Geometry: see drawing. Coordinates: mm, zero at the bounding-box minimum. Coordinates: 2 decimals unless noted, no trailing zeros. Order: outer loops, then holes, each group sorted by start corner. A loop starts at its lowest first (then second) coordinate and runs counter-clockwise, first axis right, second up. Notation, with made-up numbers: (21.5, 3) - (54.5, 3) arc R11 ccw to (54.5, 19) - close; hole circle Ø3 at (11, 8). An arc over 180 degrees is marked (long way). Use a Markdown table: item, result. Add a question column.
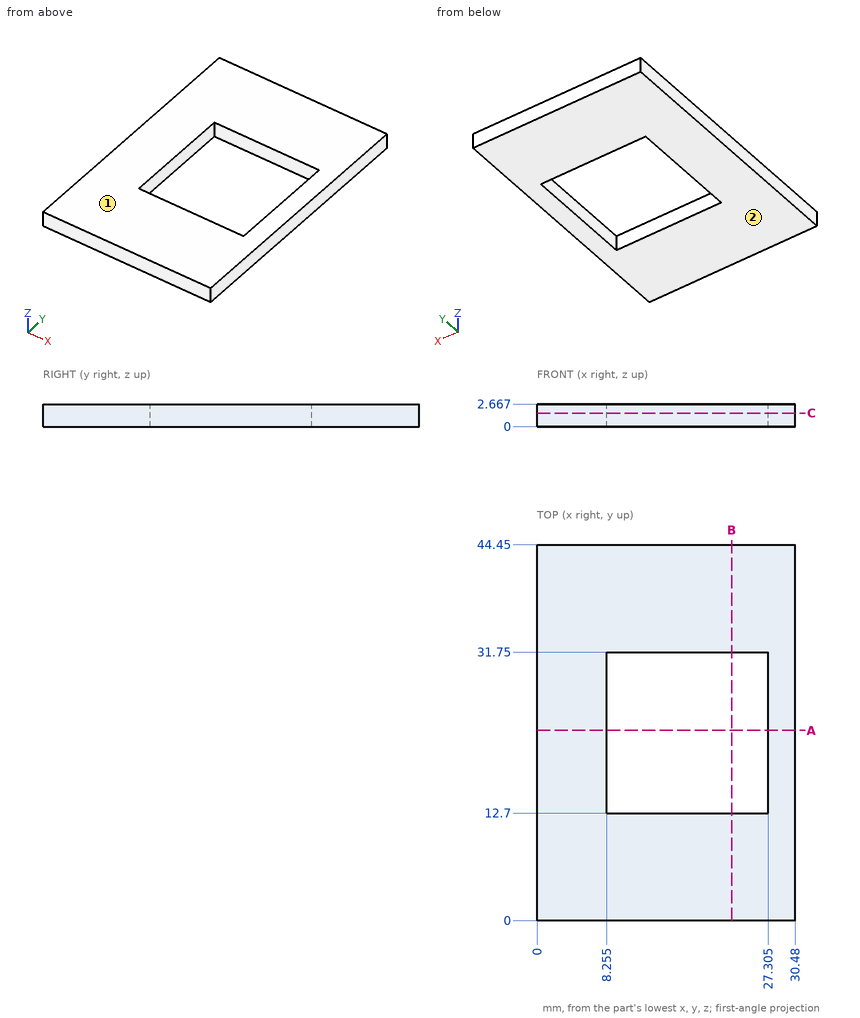
1) Section query B-B (x = 23). Return the cut outline in (y, z).
2) Line query: line 1 (Y direction, x = 14, z = 1); line 2 (X direction, y = 22, z = 1.8) (3 decimals). Output: solid intervals per line, ascending. Write a range as from..to.
3) Section query C-C (z = 1.6). Return the cut outline in (x, y) (3 decimals).
4) Section query A-A (y = 22.5). Return the cut outline in (x, z) (3 decimals), and give its area (3 significant figures).
5) Draft query along Z for the marked faces 1 and 2. Return one class per face: released by +Z, released by -Z, zero draft, split by the parting line, or undercut.
From the geometry:
| question | item | result |
|---|---|---|
| 1 | outline | (0, 0) - (12.7, 0) - (12.7, 2.67) - (0, 2.67) - close; (31.75, 0) - (44.45, 0) - (44.45, 2.67) - (31.75, 2.67) - close |
| 2 | line 1 | y = 0..12.7, 31.75..44.45 |
| 2 | line 2 | x = 0..8.255, 27.305..30.48 |
| 3 | outline | (0, 0) - (30.48, 0) - (30.48, 44.45) - (0, 44.45) - close; hole (8.255, 12.7) - (27.305, 12.7) - (27.305, 31.75) - (8.255, 31.75) - close |
| 4 | outline | (0, 0) - (8.255, 0) - (8.255, 2.667) - (0, 2.667) - close; (27.305, 0) - (30.48, 0) - (30.48, 2.667) - (27.305, 2.667) - close |
| 4 | area | 30.5 mm^2 |
| 5 | face 1 | released by +Z |
| 5 | face 2 | released by -Z |
